```python
from build123d import *

# Parameters (mm, degrees)
F0_W      = 314.325
F0_H      = 517.525
F1_DEPTH  = 369.8875
F3_DEPTH  = 200.025
F3_TAPER  = 3
F4_R      = 9.525
F5_DEPTH  = 9.525
F7_DEPTH  = 6.35
F8_R      = 5.08
F9_W      = 241.3
F9_H      = 88.9
F10_DEPTH = 1.27
F11_W     = 25.4
F11_H     = 25.4
F11_W_2   = 12.7
F12_DEPTH = 0.762


with BuildPart() as f1:
    # F0 (on Top) → F1 (new body)
    with BuildSketch(Plane.XY):
        Rectangle(F0_W, F0_H)
    extrude(amount=-F1_DEPTH)

    # F2 (on face) → F3 (cut)
    with BuildSketch(Plane.XY):
        with BuildLine():
            Line((123.825, 250.825), (-123.825, 250.825))
            ThreePointArc((-123.825, 250.825), (-141.7855122421, 243.3855122421), (-149.225, 225.425))
            Line((-149.225, 225.425), (-149.225, -225.425))
            ThreePointArc((-149.225, -225.425), (-141.7855122421, -243.3855122421), (-123.825, -250.825))
            Line((-123.825, -250.825), (123.825, -250.825))
            ThreePointArc((123.825, -250.825), (141.7855122421, -243.3855122421), (149.225, -225.425))
            Line((149.225, -225.425), (149.225, 225.425))
            ThreePointArc((149.225, 225.425), (141.7855122421, 243.3855122421), (123.825, 250.825))
        make_face()
    extrude(amount=-F3_DEPTH, taper=F3_TAPER, mode=Mode.SUBTRACT)

    # F4 (on face) → F5 (join)
    with BuildSketch(Plane(origin=(0, 0, -369.8875), x_dir=(1, 0, 0), z_dir=(0, 0, -1))):
        with Locations((-124.1987000862, 204.4887688288)):
            Circle(F4_R)
        with Locations((124.1987000862, 204.4887688288)):
            Circle(F4_R)
        with Locations((124.1987000862, -204.4887688288)):
            Circle(F4_R)
        with Locations((-124.1987000862, -204.4887688288)):
            Circle(F4_R)
    extrude(amount=F5_DEPTH)

    # F6 (on face) → F7 (join)
    with BuildSketch(Plane.XY):
        with BuildLine():
            Line((149.225, 263.525), (-149.225, 263.525))
            ThreePointArc((-149.225, 263.525), (-158.2052561211, 259.8052561211), (-161.925, 250.825))
            Line((-161.925, 250.825), (-161.925, -250.825))
            ThreePointArc((-161.925, -250.825), (-158.2052561211, -259.8052561211), (-149.225, -263.525))
            Line((-149.225, -263.525), (149.225, -263.525))
            ThreePointArc((149.225, -263.525), (158.2052561211, -259.8052561211), (161.925, -250.825))
            Line((161.925, -250.825), (161.925, 250.825))
            ThreePointArc((161.925, 250.825), (158.2052561211, 259.8052561211), (149.225, 263.525))
        make_face()
        with BuildLine():
            ThreePointArc((-149.225, 225.425), (-141.7855122421, 243.3855122421), (-123.825, 250.825))
            Line((-123.825, 250.825), (123.825, 250.825))
            ThreePointArc((123.825, 250.825), (141.7855122421, 243.3855122421), (149.225, 225.425))
            Line((149.225, 225.425), (149.225, -225.425))
            ThreePointArc((149.225, -225.425), (141.7855122421, -243.3855122421), (123.825, -250.825))
            Line((123.825, -250.825), (-123.825, -250.825))
            ThreePointArc((-123.825, -250.825), (-141.7855122421, -243.3855122421), (-149.225, -225.425))
            Line((-149.225, -225.425), (-149.225, 225.425))
        make_face(mode=Mode.SUBTRACT)
    extrude(amount=F7_DEPTH)

    # F8
    f8_edges = [f1.edges().sort_by_distance(p)[0] for p in [
        (161.925, 0, 6.35),
    ]]
    fillet(f8_edges, radius=F8_R)

    # F9 (on face) → F10 (join)
    with BuildSketch(Plane(origin=(-157.1625, 0, 0), x_dir=(0, -1, 0), z_dir=(-1, 0, 0))):
        with Locations((109.5375, -284.1625)):
            Rectangle(F9_W, F9_H)
    extrude(amount=F10_DEPTH)

    # F11 (on face) → F12 (join)
    with BuildSketch(Plane(origin=(-158.4325, 0, 0), x_dir=(0, -1, 0), z_dir=(-1, 0, 0))):
        with Locations((141.2875, -296.8625)):
            Rectangle(F11_W, F11_H)
        with Locations((160.3375, -296.8625)):
            Rectangle(F11_W_2, F11_H)
        with Locations((173.0375, -296.8625)):
            Rectangle(F11_W_2, F11_H)
        with Locations((192.0875, -296.8625)):
            Rectangle(F11_W, F11_H)
    extrude(amount=F12_DEPTH)


solid = f1.part
```
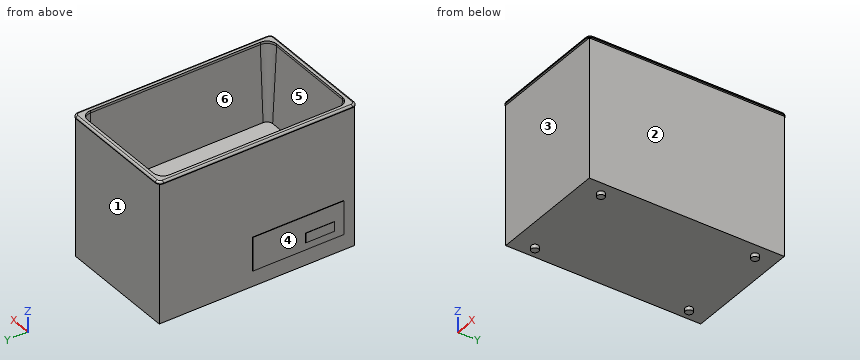
The listing builds one solid part. Answer for the finished solid, in the listing's coordinates (mm). Face numbers are marked on the shaded views. A direction names the side the tool comes from. Coordinates: 2 decimals unless noted, no trailing zeros. Write each loop counter-clockwise with the first axis right and the second up, starting at its lowest first coordinate (ties: lowest second). Pieces come first, ordered by that corner, then holes. Notation, with made-up numbers: (-39.75, -28.75) -> (-18.75, -28.75) arc R9 cw to (-18.75, -23.75) -> close; hole circle Ø4 at (44, -28.75). An arc over 180 degrees is marked (long way). Write each question's results on one line, items separated by ' | '. Start each with the question number.
1) A cutting plane is placed at D-D (z = -247). Determine the outline of the cut face in (x, y).
2) Flat-ended cylindrical pins translate along their axes: pin 1 Ø0.6 at (x, z) = (-158.5, -290.5) entering from +Y; pin 2 Ø6 at (x, y) = (-57, -79.5) entering from +Z (3 decimals); pin 3 Ø1.9 at (x, z) = (36, 3) entering from -Y. Find the tip coordinate at first contact, or state that the pin passes through.
3) Straight lines are drawn through the part: probe 1 along X at (y, z) = (86, -270); probe 2 along Z at (x, y) = (-87, -75) (1 decimal); probe 3 along X at (y, z) = (102.5, -8.5). For each, find the intervals that lie inside material, in ascending order.
4) A cutting plane is placed at B-B (z = -65). Determine the outline of the cut face in (x, y) (1 decimal), then the cut area to 3 significant figures.
5) For a pull along Y with two mould halves and no side action, classify the marked faces 3, 4, 5 and 6 as +Y half, -Y half, draft (parallel to the pull), parting line (faces both ways), or undercut.
6) A tool of negligible diameter and unlimited length cuts with its end or side. For the marked faces 1 and 2, from which of +Z, -Z, +X, -X, +Y, -Y can it reach the whole face along a straight path? Write none if from no direction.
Values follow:
1) outline: (-158.43, -230.19) -> (-157.16, -230.19) -> (-157.16, -258.76) -> (157.16, -258.76) -> (157.16, 258.76) -> (-157.16, 258.76) -> (-157.16, 11.11) -> (-158.43, 11.11) -> close
2) pin 1: y = 11.11 | pin 2: z = -200.025 | pin 3: y = -263.46
3) probe 1: -157.16 to 157.16 | probe 2: -369.9 to -200 | probe 3: -157.16 to -148.78, 148.78 to 157.16
4) outline: (-157.2, -258.8) -> (157.2, -258.8) -> (157.2, 258.8) -> (-157.2, 258.8) -> close; hole (-145.8, -225.4) arc R22 ccw to (-123.8, -247.4) -> (123.8, -247.4) arc R22 ccw to (145.8, -225.4) -> (145.8, 225.4) arc R22 ccw to (123.8, 247.4) -> (-123.8, 247.4) arc R22 ccw to (-145.8, 225.4) -> close | area: 18,800 mm²
5) face 3: -Y half | face 4: draft | face 5: undercut | face 6: undercut
6) face 1: -Z, +X, -X, +Y | face 2: -Z, +X, +Y, -Y
